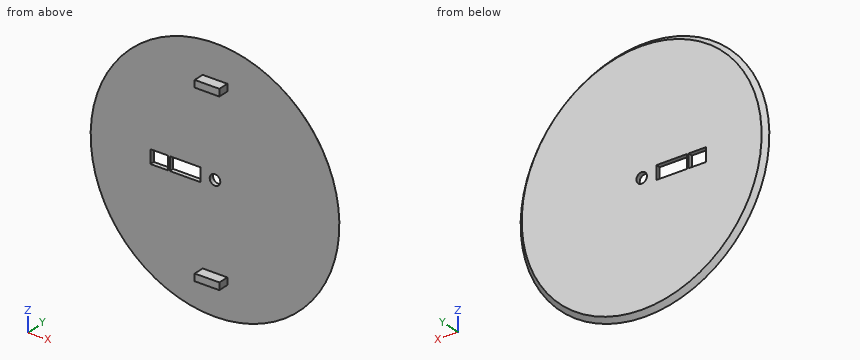
from build123d import *

# Parameters (mm, degrees)
FRONT_W                                  = 21.45
FRONT_H                                  = 0.75
SKETCH1_W                                = 4.2
SKETCH1_H                                = 1.2
HOLDERS_DEPTH                            = 1.8
HOLES_START                              = -0.375
HOLES_MOUNT_CALENDAR_PATTERN_OUTLINE_W   = 3
HOLES_MOUNT_CALENDAR_PATTERN_OUTLINE_H   = 2.3
HOLES_MOUNT_CALENDAR_PATTERN_OUTLINE_W_2 = 5.2
HOLES_MOUNT_CALENDAR_PATTERN_OUTLINE_R   = 0.9
HOLES_MOUNT_CALENDAR_PATTERN_DEPTH       = 0.75
CHAMFER1_SIZE                            = 1


# Read off the part's stored shape, not the designer's step: Holes Mount & Calendar & Pattern
with BuildPart() as part:
    # Front → Base (revolve)
    with BuildSketch(Plane.XY, mode=Mode.PRIVATE) as base_sk:
        with Locations((-10.725, 0)):
            Rectangle(FRONT_W, FRONT_H)
    revolve(base_sk.sketch.rotate(Axis((0, 0, 0), (0, 1, 0)), 270), axis=Axis((0, 0, 0), (0, 1, 0)))

    # Sketch1 → Holders (add)
    with BuildSketch(Plane.XZ.offset(0.375)):
        with Locations((0, 15)):
            Rectangle(SKETCH1_W, SKETCH1_H)
        with Locations((0, -15)):
            Rectangle(SKETCH1_W, SKETCH1_H)
    extrude(amount=HOLDERS_DEPTH)

    # Holes Mount & Calendar & Pattern outline → Holes Mount & Calendar & Pattern (cut)
    with BuildSketch(Plane(origin=(0, 0, 0), x_dir=(1, 0, 0), z_dir=(0, 1, 0)).offset(HOLES_START)):
        with Locations((-9.5, 0)):
            Rectangle(HOLES_MOUNT_CALENDAR_PATTERN_OUTLINE_W, HOLES_MOUNT_CALENDAR_PATTERN_OUTLINE_H)
        with Locations((-5.1, 0)):
            Rectangle(HOLES_MOUNT_CALENDAR_PATTERN_OUTLINE_W_2, HOLES_MOUNT_CALENDAR_PATTERN_OUTLINE_H)
        Circle(HOLES_MOUNT_CALENDAR_PATTERN_OUTLINE_R)
    extrude(amount=HOLES_MOUNT_CALENDAR_PATTERN_DEPTH, mode=Mode.SUBTRACT)

    # Chamfer1
    # the kernel refuses this chamfer: 1 mm, written as the material it takes off along each edge
    with BuildSketch(Plane(origin=(0, 0.375, 0), x_dir=(0, 0, -1), z_dir=(1, 0, 0))) as chamfer1_piece_1:
        Polygon((21.45, -CHAMFER1_SIZE), (21.45 - CHAMFER1_SIZE, 0), (21.45, 0), align=None)
    revolve(axis=Axis((0, 0.375, 0), (0, 1, 0)), mode=Mode.SUBTRACT)


solid = part.part
Check sheet for the modelled part. Datum: model origin and axes. Units: mm. Give positions to 0.01 mm unless a question says otherwise; leave off trailing zeros. Loops run counter-clockwise (first coordinate to the right, second up) from the corner with the lowest first, then second, coordinate; pieces in that order, holes last. Notation, with made-up numbers: M 46.25,58.5 L 94.25,58.5 A22 ccw 94.25,88.5 Z; hole C -38,57.5 d7. An arc over 180 degrees is marked long. Use a Markdown table: item, result. Add a question column.
Q1. Sectioned sample at B-B, the plane z = 0. Record the cut outline in (x, y) (3 decimals).
Q2. Sectioned sample at A-A, the plane x = 0. Record the cut outline in (y, z) (3 decimals).
Q3. Go/stop test with flat-tipped pins: pin 1 (0.6 mm diameter, centred on x = -4.5, y = 0, fed in from -Z); pin 2 (1 mm diameter, centred on y = -1, z = 15, fed in from +X); pin 3 (1.5 mm diameter, centred on x = 3.5, y = -1, fed in from +Z). Record where each tip stops, or that it passes through.
Q4. Scan lines: line 1 along Z through (x, y) = (2, -1.85); line 2 along X through (y, z) = (0, 0) (3 decimals); line 3 along Z through (x, y) = (0, 0.15) (3 decimals). Record each from-to range of solid material in increasing order. Write a range as [from, to].
Verdict:
| question | item | result |
|---|---|---|
| 1 | outline | M -21.2,-0.375 L -11,-0.375 L -11,0.375 L -20.45,0.375 Z; M -8,-0.375 L -7.7,-0.375 L -7.7,0.375 L -8,0.375 Z; M -2.5,-0.375 L -0.9,-0.375 L -0.9,0.375 L -2.5,0.375 Z; M 0.9,-0.375 L 21.2,-0.375 L 20.45,0.375 L 0.9,0.375 Z |
| 2 | outline | M -2.175,-15.6 L -0.375,-15.6 L -0.375,-21.2 L 0.375,-20.45 L 0.375,-0.9 L -0.375,-0.9 L -0.375,-14.4 L -2.175,-14.4 Z; M -2.175,14.4 L -0.375,14.4 L -0.375,0.9 L 0.375,0.9 L 0.375,20.45 L -0.375,21.2 L -0.375,15.6 L -2.175,15.6 Z |
| 3 | pin 1 | z = -20.65 |
| 3 | pin 2 | x = 2.1 |
| 3 | pin 3 | z = 20.97 |
| 4 | line 1 | [-15.6, -14.4], [14.4, 15.6] |
| 4 | line 2 | [-20.825, -11], [-8, -7.7], [-2.5, -0.9], [0.9, 20.825] |
| 4 | line 3 | [-20.675, -0.9], [0.9, 20.675] |
